```python
from build123d import *

# Parameters (mm, degrees)
SKETCH1_W           = 140
SKETCH1_H           = 70
BOSS_EXTRUDE1_DEPTH = 19
SKETCH2_W           = 38.1
SKETCH2_H           = 9
BOSS_EXTRUDE2_DEPTH = 70
SKETCH3_R           = 9.5
CUT_EXTRUDE1_DEPTH  = 84.120394609
SKETCH4_R           = 35
SKETCH4_R_2         = 19.05
BOSS_EXTRUDE3_DEPTH = 51
BOSS_EXTRUDE4_DEPTH = 22
RIB5_REACH          = 169.419
SKETCH10_WALL_W     = 398.82114278
SKETCH10_WALL_H     = 19


with BuildPart() as part:
    # Sketch1 → Boss-Extrude1 (new body)
    with BuildSketch(Plane(origin=(0, 0, 0), x_dir=(1, 0, 0), z_dir=(0, 1, 0))):
        Rectangle(SKETCH1_W, SKETCH1_H)
    extrude(amount=BOSS_EXTRUDE1_DEPTH)

    # Sketch2 → Boss-Extrude2 (add)
    with BuildSketch(Plane.XY.offset(35)):
        with Locations((0, -4.5)):
            Rectangle(SKETCH2_W, SKETCH2_H)
    extrude(amount=-BOSS_EXTRUDE2_DEPTH)

    # Sketch3 → Cut-Extrude1 (cut, through all)
    with BuildSketch(Plane(origin=(0, 19, 0), x_dir=(1, 0, 0), z_dir=(0, 1, 0))):
        with Locations(Location((41, -10, 0), (0, 0, 270))):
            Circle(SKETCH3_R)
        with Locations(Location((-41, -10, 0), (0, 0, 270))):
            Circle(SKETCH3_R)
    extrude(amount=-CUT_EXTRUDE1_DEPTH, mode=Mode.SUBTRACT)



with BuildPart() as body_2:
    # Sketch4 → Boss-Extrude3 (new body)
    with BuildSketch(Plane(origin=(0, 0, -35), x_dir=(-1, 0, 0), z_dir=(0, 0, -1))):
        with Locations((0, 113)):
            Circle(SKETCH4_R)
        with Locations((0, 113)):
            Circle(SKETCH4_R_2, mode=Mode.SUBTRACT)
    extrude(amount=-BOSS_EXTRUDE3_DEPTH)


with BuildPart() as part_1:
    add(part.part)

    add(body_2.part)  # Boss-Extrude4 merges body 2
    # Sketch7 → Boss-Extrude4 (add)
    with BuildSketch(Plane(origin=(0, 0, -35), x_dir=(-1, 0, 0), z_dir=(0, 0, -1))):
        with BuildLine():
            Line((-70, 19), (-33.033269752, 124.567328538))
            ThreePointArc((-33.033269752, 124.567328538), (0, 78), (33.033269752, 124.567328538))
            Line((33.033269752, 124.567328538), (70, 19))
            Line((70, 19), (-70, 19))
        make_face()
    extrude(amount=-BOSS_EXTRUDE4_DEPTH)

    # Sketch10 wall → Rib5 (add, up to next)
    with BuildSketch(Plane(origin=(0, 48.5, 25.5), x_dir=(0, 0.951860557857, -0.306531366089), z_dir=(0, 0.306531366089, 0.951860557857)), mode=Mode.PRIVATE) as rib5_sk1:
        Rectangle(SKETCH10_WALL_W, SKETCH10_WALL_H)
    rib5_tool1 = extrude(rib5_sk1.sketch, amount=-RIB5_REACH, mode=Mode.PRIVATE) - part_1.part
    add(rib5_tool1.solids().sort_by_distance((0, 48.5, 25.5))[0])


solid = part_1.part
```
Geometry: final body of the model. Coordinates: model frame, mm. A direction names the side the tool comes from. Round coordinates to 2 decimals unless told otherwise and drop trailing zeros. Order: outer loops, then holes, each group sorted by start corner. A loop starts at its lowest first (then second) coordinate and runs counter-clockwise, first axis right, second up. Notation, with made-up numbers: (16.5, 23.5) - (43.5, 23.5) arc R17 ccw to (43.5, 42.5) - close; hole circle Ø4 at (-19.5, 17.25). An arc over 180 degrees is marked (long way). Write item = value, one per line. Start each with the question number.
Q1. Cut plane C-C on x = -21. Return the cut outline in (y, z).
Q2. Cut plane B-B on z = -26.5. Return the cut outline in (x, y).
Q3. Ray query, line 1 (X direction, y = 6, z = 10); line 2 (Y direction, x = 12, z = -9); line 3 (Y direction, x = 0, z = -15). Return the intervals inside material, ascending. Write a range as from..to.
Q4. Cut plane A-A on z = 10. Return the cut outline in (x, y).
Q5. Access query for faces 1 (the flat face through (-15, 98, 16)), 2 (the cylindrical face through (-32.99, 9.63, 15.11)), 3 (the flat face through (19.05, -5, 0)), 4 (the flat face through (-33, 49, -13)), 5 (the flat face through (9.5, 47, 7)). Directions: +Z, -Z, +X, -X, +Y, -Y. A direction counts if a zero-diameter tool reaches every point of the face in a straight line with its end or side. Return the directions, or none.
Q6. Pull-direction query (Y, two-part tool) for faces 6 (the flat face through (-70, 9, 0)), 7 (the flat face through (0, -9, 0)), 8 (the flat face through (33, 49, -13)); classes: +Y half, -Y half, draft (parallel to the pull), parting line (faces both ways), or undercut.
Q7. Cut plane D-D on y = 102. Return the cut outline in (x, z), and give its area (3 significant figures).
Q8. Pin query (flat end, axial travel): pin 1 (15.5 mm diameter, centred on x = 34.5, z = -15, fed in from -Y); pin 2 (12 mm diameter, centred on x = 26, y = 74, fed in from +Z); pin 3 (14.5 mm diameter, centred on y = 35.5, z = 8.5, fed in from -X); pin 4 (11.5 mm diameter, centred on x = 41, z = 10, fed in from +Y). Return the tip coordinate at first contact, or that it passes through.
Outcome:
q1.outline = (0, -35) - (141, -35) - (141, 16) - (85, 16) - (85, -13) - (19, -13) - (19, 35) - (0, 35) - close
q2.outline = (-70, 0) - (-19.05, 0) - (-19.05, -9) - (19.05, -9) - (19.05, 0) - (70, 0) - (70, 19) - (33.03, 124.57) arc R35 ccw to (-33.03, 124.57) - (-70, 19) - close; hole circle Ø38.1 at (0, 113)
q3.line_1 = -70..-50.5, -31.5..31.5, 50.5..70
q3.line_2 = -9..19, 80.12..98.2, 127.8..145.88
q3.line_3 = -9..93.95, 132.05..148
q4.outline = (-70, 0) - (-50.5, 0) - (-50.5, 19) - (-70, 19) - close; (-31.5, 0) - (-19.05, 0) - (-19.05, -9) - (19.05, -9) - (19.05, 0) - (31.5, 0) - (31.5, 19) - (9.5, 19) - (9.5, 79.31) arc R35 ccw (long way) to (-9.5, 79.31) - (-9.5, 19) - (-31.5, 19) - close; (50.5, 0) - (70, 0) - (70, 19) - (50.5, 19) - close; hole circle Ø38.1 at (0, 113)
q5.face_1 = +Z, +X, -X, +Y
q5.face_2 = -Y
q5.face_3 = +Z, -Z, +X, -Y
q5.face_4 = +Z, -X
q5.face_5 = +Z, +X
q6.face_6 = draft
q6.face_7 = -Y half
q6.face_8 = undercut
q7.outline = (-40.94, -35) - (-15.55, -35) - (-15.55, 16) - (-33.23, 16) - (-33.23, -13) - (-40.94, -13) - close; (15.55, -35) - (40.94, -35) - (40.94, -13) - (33.23, -13) - (33.23, 16) - (15.55, 16) - close
q7.area = 2,140 mm^2
q8.pin_1 = 0
q8.pin_2 = -13
q8.pin_3 = -9.5
q8.pin_4 = through
